```python
from build123d import *

# Parameters (mm, degrees)
F0_W     = 85
F0_H     = 126
F1_DEPTH = 65
F3_DEPTH = 200
F5_DEPTH = 100


with BuildPart() as f1:
    # F0 (on Front) → F1 (new body)
    with BuildSketch(Plane.XZ):
        Rectangle(F0_W, F0_H)
    extrude(amount=F1_DEPTH)

    # F2 (on face) → F3 (cut)
    with BuildSketch(Plane.XY.offset(63)):
        with BuildLine():
            ThreePointArc((42.5, 0), (39.220219, -13.260584), (30.137157, -23.463428))
            ThreePointArc((30.137157, -23.463428), (23.716021, -26.537316), (16.649198, -27.397415))
            ThreePointArc((16.649198, -27.397415), (10.926292, -33.802126), (15.103702, -41.306872))
            ThreePointArc((15.103702, -41.306872), (25.834637, -53.153436), (15.103702, -65))
            Line((15.103702, -65), (42.5, -65))
            Line((42.5, -65), (42.5, 0))
        make_face()
    extrude(amount=-F3_DEPTH, mode=Mode.SUBTRACT)

    # F4 (on face) → F5 (cut)
    with BuildSketch(Plane(origin=(-42.5, 0, 0), x_dir=(0, -1, 0), z_dir=(-1, 0, 0))):
        Polygon((65, 63), (0, 63), (25.149422, 50.228592), (65, 45.170609), align=None)
    extrude(amount=-F5_DEPTH, mode=Mode.SUBTRACT)


solid = f1.part
```
Design review of the part built by this model. Coordinates are the model's own, in mm. Coordinates: 2 decimals unless noted, no trailing zeros. Order: outer loops, then holes, each group sorted by start corner. A loop starts at its lowest first (then second) coordinate and runs counter-clockwise, first axis right, second up. Notation, with made-up numbers: (15, 76) -> (65, 76) arc R22 ccw to (65, 100) -> close; hole circle Ø10 at (10, 70.5). An arc over 180 degrees is marked (long way). One line per item, written item: value. Start each with the question number.
Q1. Take a section at D-D, the plane y = -11. State the section outline as (x, z) points, then the cut area to 3 significant figures.
Q2. Mouldability with a two-part tool opening along Y and no side actions: class faces 1 (the flat face through (-8.097, -44.796, 47.735)), 2 (the flat face through (-1, 0, 1)), 3 (the cylindrical face through (25.832, -52.908, -6.633)) as pulls with the +Y half, pulls with the -Y half, needs draft (parallel to the pull), parting line crosses it, or undercut.
Q3. Take a section at B-B, the plane x = -24. State the section outline as (y, z) points, then the cut area to 3 significant figures.
Q4. Take a section at A-A, the plane z = -45. State the section outline as (x, y) points, then the cut area to 3 significant figures.
Q5. Insertion check: pin 1 Ø6 at (x, y) = (-2.5, -24) entering from +Z; pin 2 Ø8 at (x, y) = (14.5, -52.5) entering from +Z; pin 3 Ø6 at (y, z) = (-49, -2) entering from +X. Each pin has a flat end and moves straight along its axis. Give the tip position at first contact, or say it passes through.
Q6. Take a section at C-C, the plane y = -57. State the section outline as (x, z) points.
Q7. For probe 1 along X at (y, z) = (-53, -54); probe 2 along X at (y, z) = (-34, -27.5); probe 3 along Y at (x, z) = (23.5, -46.5), list the stretches that pass through material, from the lowest coordinate up.
Values follow:
1. outline: (-42.5, -63) -> (40.29, -63) -> (40.29, 57.41) -> (-42.5, 57.41) -> close
1. area: 9,970 mm2
2. face 1: pulls with the -Y half
2. face 2: pulls with the +Y half
2. face 3: undercut
3. outline: (-65, -63) -> (0, -63) -> (0, 63) -> (-25.15, 50.23) -> (-65, 45.17) -> close
3. area: 7,420 mm2
4. outline: (-42.5, -65) -> (15.1, -65) arc R11.9 ccw to (15.1, -41.31) arc R7.41 cw to (16.65, -27.4) arc R21.98 ccw to (30.14, -23.46) arc R28.45 ccw to (42.5, 0) -> (-42.5, 0) -> close
4. area: 4,500 mm2
5. pin 1: stops at z = 52.34
5. pin 2: stops at z = 47.26
5. pin 3: stops at x = 25.78
6. outline: (-42.5, -63) -> (25.2, -63) -> (25.2, 46.19) -> (-42.5, 46.19) -> close
7. probe 1: x = -42.5 to 25.83
7. probe 2: x = -42.5 to 10.91
7. probe 3: y = -60.23 to -46.07, -26.6 to 0
